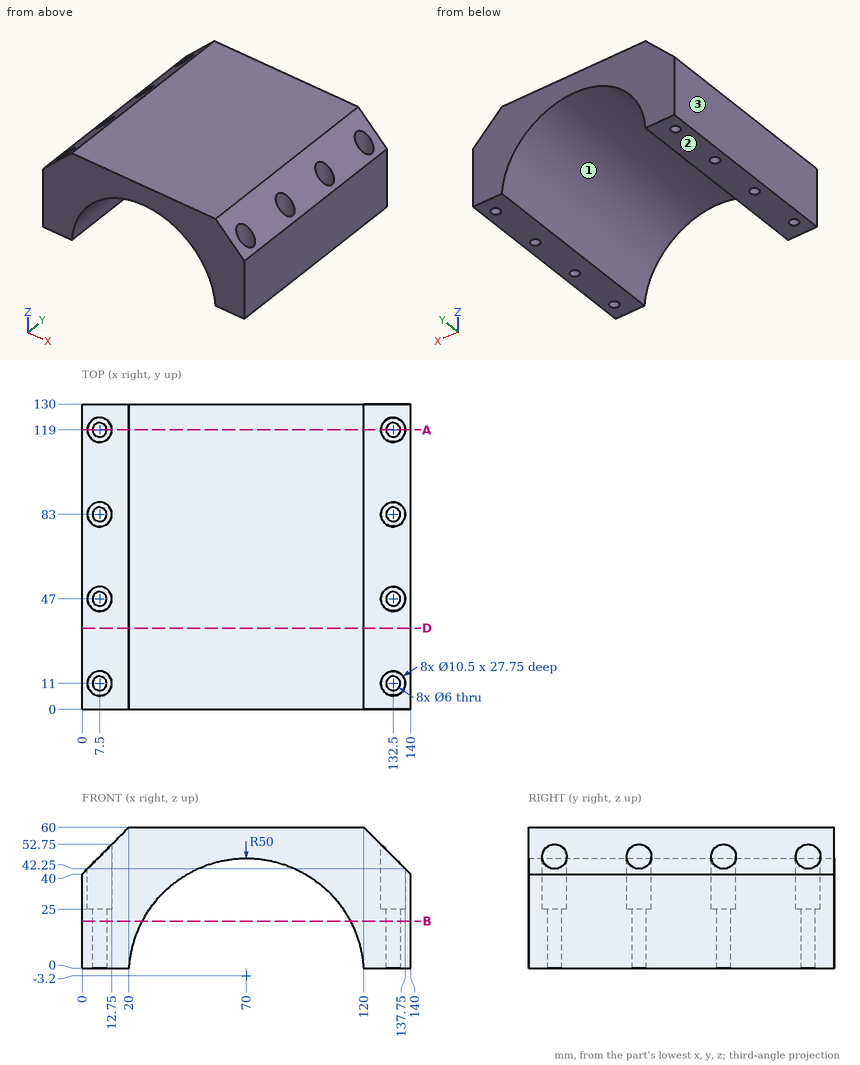
Input: dimensioned drawing with shaded views. Units: mm. Origin: part minimum x, y, z. Coordinates: 2 decimals unless noted, no trailing zeros. Loops run counter-clockwise (first coordinate to the right, second up) from the corner with the lowest first, then second, coordinate; pieces in that order, holes last. Notation, with made-up numbers: M -4,10 L 29,10 A18 ccw 29,30 Z; hole C 65.25,57.5 d9. An arc over 180 degrees is marked long. One line per item, written item: value. Start each with the question number.
1) Cut plane B-B (z = 20). Count the separate pieces of the cut face and the enclosed holes in it, then the cut area to 3 significant figures.
2) Material intervals for L1, parallel to Y at x = 7, z = 33; L2, parallel to Y at x = 132.5, z = 8; L3, parallel to X at y = 80.5, z = 22.5, sorted ascending. Write a range as from..to.
3) Cut plane A-A (y = 119). Return loops of the section in (x, z).
4) Cut plane D-D (y = 34.5). Return loops of the section in (x, z).
5) Draft query along X for the marked faces 1, 2 and 3. Return one class per face: released by +X, released by -X, zero draft, split by the parting line, or undercut.
6) Pin query (flat end, axial travel): P1, Ø11.5, axis at x = 8.5, y = 47, coming from the +Z side; P2, Ø8, axis at x = 132.5, y = 47, coming from the +Z side; P3, Ø11.5, axis at x = 133, y = 49, coming from the +Z side. Return the tip coordinate at first contact, or that it passes through.
Evaluation:
1. separate pieces: 2
1. enclosed holes: 8
1. area: 6,460 mm^2
2. L1: 0..5.77, 16.23..41.77, 52.23..77.77, 88.23..113.77, 124.23..130
2. L2: 0..8, 14..44, 50..80, 86..116, 122..130
2. L3: 0..5.84, 9.16..27.11, 112.89..130.84, 134.16..140
3. outline: M 0,0 L 4.5,0 L 4.5,25 L 2.25,25 L 2.25,42.25 L 0,40 Z; M 10.5,0 L 20.1,0 A50 cw 119.9,0 L 129.5,0 L 129.5,25 L 127.25,25 L 127.25,52.75 L 120,60 L 20,60 L 12.75,52.75 L 12.75,25 L 10.5,25 Z; M 135.5,0 L 140,0 L 140,40 L 137.75,42.25 L 137.75,25 L 135.5,25 Z
4. outline: M 0,0 L 20.1,0 A50 cw 119.9,0 L 140,0 L 140,40 L 120,60 L 20,60 L 0,40 Z
5. face 1: undercut
5. face 2: zero draft
5. face 3: released by -X
6. P1: z = 54.25
6. P2: z = 25
6. P3: z = 52.75
